Geometry: see drawing. Coordinates: mm, zero at the bounding-box minimum. A direction names the side the tool comes from. Give positions to 0.01 mm unless a question says otherwise; leave off trailing zeros. Write each loop counter-clockwise with the first axis right and the second up, starting at its lowest first coordinate (ties: lowest second). Pieces come first, ordered by that corner, then holes. Notation, with made-up numbers: (-8.75, 83) -> (13.25, 83) arc R19 cw to (13.25, 114) -> close; hole circle Ø5 at (75, -11). An arc over 180 degrees is marked (long way). Use one line per item in the form item = value. Start each with the question number.
(1) Set-up query: the marked faces 1 and 2. Return all of +Z, -Z, +X, -X, +Y, -Y with unobstructed straight access to the full face (end or side cutting, diameter ignored); none if empty.
(2) First-contact query: P1, Ø7, axis at x = 214, z = 239.5, coming from the -Y side; P2, Ø5, axis at x = 104, y = 81, coming from the +Z side; P3, Ø7, axis at x = 87, z = 220.5, coming from the +Y side. Flat tips, straight axial feed; report the tip coordinate or a pass-through.
(3) Cut plane B-B, the plane y = 35. Output: boundary loops of the cut face in (x, z).
(4) Cut plane A-A, the plane z = 247. Output: boundary loops of the cut face in (x, y).
(5) Cut plane C-C, the plane x = 157. Output: boundary loops of the cut face in (y, z).
(6) Draft query along Z for the marked faces 3, 4 and 5. Return one class per face: pulls with the +Z half, pulls with the -Z half, needs draft (parallel to the pull), parting line crosses it, or undercut.
(7) Material intervals for line 1 along X through (y, z) = (129, 11); line 2 along Z through (x, y) = (149.5, 17.5); line 3 along Z through (x, y) = (197, 169), sorted ascending. Write a range as from..to.
(8) Cut plane D-D, the plane y = 89.5. Output: boundary loops of the cut face in (x, z).
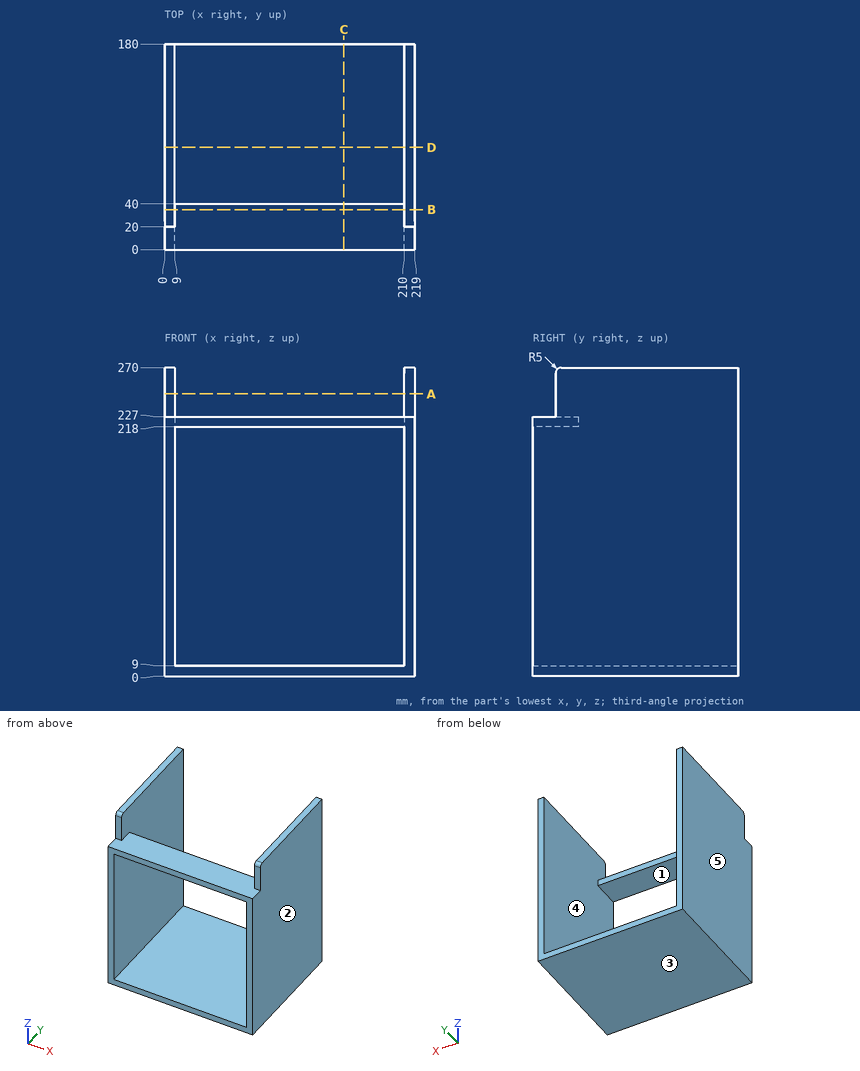
Geometry says:
q1.face_1 = +Y, -Y
q1.face_2 = +Z, -Z, +X, +Y, -Y
q2.P1 = 20
q2.P2 = 9
q2.P3 = 40
q3.outline = (0, 0) -> (219, 0) -> (219, 270) -> (210, 270) -> (210, 227) -> (9, 227) -> (9, 270) -> (0, 270) -> close; hole (9, 9) -> (210, 9) -> (210, 218) -> (9, 218) -> close
q4.outline = (0, 20) -> (9, 20) -> (9, 180) -> (0, 180) -> close; (210, 20) -> (219, 20) -> (219, 180) -> (210, 180) -> close
q5.outline = (0, 0) -> (180, 0) -> (180, 9) -> (0, 9) -> close; (0, 218) -> (40, 218) -> (40, 227) -> (0, 227) -> close
q6.face_3 = pulls with the -Z half
q6.face_4 = undercut
q6.face_5 = needs draft
q7.line_1 = 0..9, 210..219
q7.line_2 = 0..9, 218..227
q7.line_3 = 0..9
q8.outline = (0, 0) -> (219, 0) -> (219, 270) -> (210, 270) -> (210, 9) -> (9, 9) -> (9, 270) -> (0, 270) -> close
